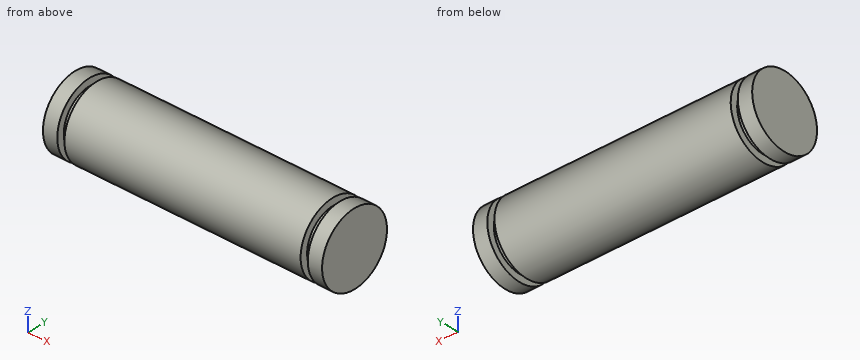
```python
from build123d import *


with BuildPart() as part:
    # Sketch2 → Revolve1 (revolve)
    with BuildSketch(Plane.XY):
        Polygon((0, 2.5), (0, 0), (-19.5, 0), (-19.5, 2.5), (-18.5, 2.5), (-18.5, 2), (-18, 2), (-18, 2.5), (-1.5, 2.5), (-1.5, 2), (-1, 2), (-1, 2.5), align=None)
    revolve(axis=Axis((0, 0, 0), (-1, 0, 0)))


solid = part.part
```
Model file for the job. Use its own axes, mm. Coordinates: 2 decimals unless noted, no trailing zeros. Order: outer loops, then holes, each group sorted by start corner. A loop starts at its lowest first (then second) coordinate and runs counter-clockwise, first axis right, second up. Notation, with made-up numbers: (-2.5, 33.25) - (11.5, 33.25) arc R20 ccw to (11.5, 71.25) - close; hole circle Ø7 at (85.5, 1). An arc over 180 degrees is marked (long way). Return JSON: item names as keys, results as strings. Group by question number.
1) Saw through at A-A, the plane z = 0.6. Write the cut outline in (x, y), plus the area to 3 significant figures.
2) Saw through at B-B, the plane y = 0.55. Write the cut outline in (x, z).
3) Flat gauge pin, fed straight in: P1, Ø1, axis at y = 1, z = -1, coming from the +X side. Where does the tip first touch, or does it go through?
4) Saw through at C-C, the plane x = -14.75. Write the cut outline in (y, z), plus the area to 3 significant figures.
5) Probe line 1 (X direction, y = -2, z = -0.6); line 2 (Y direction, x = -2, z = 1.5); line 3 (Z direction, x = -7.75, y = -0.1). List the from-to ranges inside material, lowest first. Write a range as from..to.
Values found:
{
 "1": {"outline": "(-19.5, -2.43) - (-18.5, -2.43) - (-18.5, -1.91) - (-18, -1.91) - (-18, -2.43) - (-1.5, -2.43) - (-1.5, -1.91) - (-1, -1.91) - (-1, -2.43) - (0, -2.43) - (0, 2.43) - (-1, 2.43) - (-1, 1.91) - (-1.5, 1.91) - (-1.5, 2.43) - (-18, 2.43) - (-18, 1.91) - (-18.5, 1.91) - (-18.5, 2.43) - (-19.5, 2.43) - close", "area": "93.6 mm²"},
 "2": {"outline": "(-19.5, -2.44) - (-18.5, -2.44) - (-18.5, -1.92) - (-18, -1.92) - (-18, -2.44) - (-1.5, -2.44) - (-1.5, -1.92) - (-1, -1.92) - (-1, -2.44) - (0, -2.44) - (0, 2.44) - (-1, 2.44) - (-1, 1.92) - (-1.5, 1.92) - (-1.5, 2.44) - (-18, 2.44) - (-18, 1.92) - (-18.5, 1.92) - (-18.5, 2.44) - (-19.5, 2.44) - close"},
 "3": {"P1": "stops at x = 0"},
 "4": {"outline": "circle Ø5 at (0, 0)", "area": "19.6 mm²"},
 "5": {"line 1": "x = -19.5..-18.5, -18..-1.5, -1..0", "line 2": "y = -2..2", "line 3": "z = -2.5..2.5"}
}
